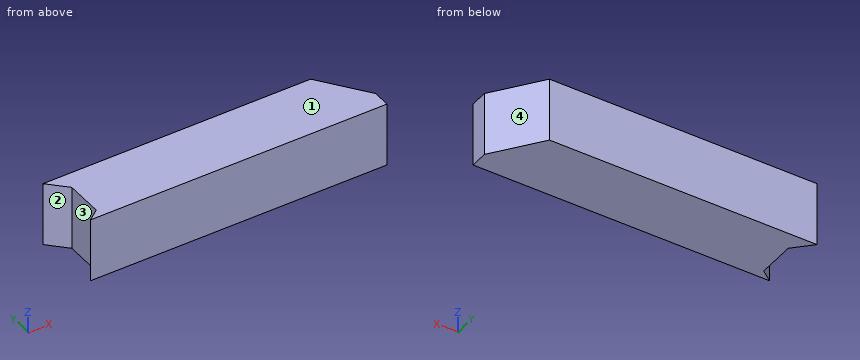
```python
from build123d import *

# Parameters (mm, degrees)
F0_W     = 5.5
F0_H     = 5.5
F1_DEPTH = 13
F3_DEPTH = 5.501


with BuildPart() as f1:
    # F0 (on Right) → F1 (new body, symmetric)
    with BuildSketch(Plane.YZ):
        with Locations((2.75, -2.75)):
            Rectangle(F0_W, F0_H)
    extrude(amount=F1_DEPTH, both=True)

    # F2 (on face) → F3 (cut, through all)
    with BuildSketch(Plane.XY):
        Polygon((-11.5, 4), (-13, 5.5), (-13, 0), (-12.5, 0), (-11.5, 0.75), align=None)
        Polygon((13, 5.5), (10, 5.5), (13, 1.5), align=None)
    extrude(amount=-F3_DEPTH, mode=Mode.SUBTRACT)


solid = f1.part
```
The listing builds one solid part. Answer for the finished solid, in the listing's coordinates (mm). Face numbers are marked on the shaded views. Give positions to 0.01 mm unless a question says otherwise; leave off trailing zeros. Order: outer loops, then holes, each group sorted by start corner. A loop starts at its lowest first (then second) coordinate and runs counter-clockwise, first axis right, second up. Notation, with made-up numbers: (36, -36.75) -> (86, -36.75) arc R31 ccw to (86, -1.75) -> close; hole circle Ø8 at (46, 81.5). An arc over 180 degrees is marked (long way). Answer as a JSON object with one key per item and string values. Group by question number.
Item 1: A flat-ended cylindrical pin translates along its axis: pin 1 (3 mm diameter, centred on y = 0.5, z = -2.5, fed in from -X). Find the tip coordinate at first contact, or state that the pin passes through.
Item 2: Consider L1, parallel to X at y = 0.9, z = -1.75; L2, parallel to X at y = 3, z = -2.05 (3 decimals). Determine where each line is inside the solid, lowest interval first. Write a range as from..to.
Item 3: The part is cut by section A-A on z = -0.4. Write down the section's boundary in (x, y).
Item 4: Determine the mould class of the marked faces 1, 2, 3 and 4 for opening direction Y: pulls with the +Y half, pulls with the -Y half, needs draft (parallel to the pull), parting line crosses it, or undercut.
Item 5: The part is cut by section C-C on x = 11. Write down the section's boundary in (y, z), and give its area (3 significant figures).
Item 6: The part is cut by section B-B on y = 1.2. Write down the section's boundary in (x, z), and give its area (3 significant figures).
Result set:
{
 "1": {"pin 1": "x = -12.5"},
 "2": {"L1": "-11.5..13", "L2": "-11.5..11.875"},
 "3": {"outline": "(-13, 5.5) -> (-11.5, 4) -> (-11.5, 0.75) -> (-12.5, 0) -> (13, 0) -> (13, 1.5) -> (10, 5.5) -> close"},
 "4": {"face 1": "needs draft", "face 2": "undercut", "face 3": "undercut", "face 4": "pulls with the +Y half"},
 "5": {"outline": "(0, -5.5) -> (4.17, -5.5) -> (4.17, 0) -> (0, 0) -> close", "area": "22.9 mm²"},
 "6": {"outline": "(-11.5, -5.5) -> (13, -5.5) -> (13, 0) -> (-11.5, 0) -> close", "area": "135 mm²"}
}
